Can you work these out from the model? Positions are in its coordinate system, mm. Face numbers are marked on the shaded views. A direction names the side the tool comes from. Give positions to 0.01 mm unless a question says otherwise; leave off trailing zeros. Loops run counter-clockwise (first coordinate to the right, second up) from the corner with the lowest first, then second, coordinate; pieces in that order, holes last.
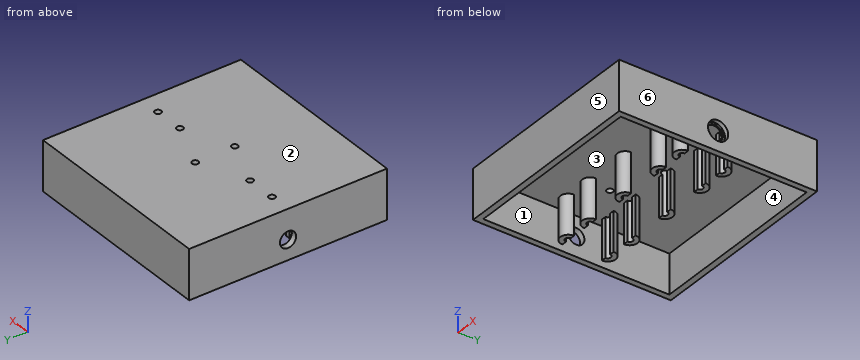
from build123d import *

# Parameters (mm, degrees)
F0_W           = 100
F0_H           = 100
F1_DEPTH       = 25
F2_W           = 94
F2_H           = 94
F3_DEPTH       = 20
F5_D           = 8.2
F5_CBORE_D     = 10.2
F5_CBORE_DEPTH = 2.2
F6_R           = 4
F7_DEPTH       = 25
F9_D           = 3.2
F10_R          = 1.6
F11_DEPTH      = 20
F12_W          = 94
F12_H          = 20
F13_DEPTH      = 20


with BuildPart() as f1:
    # F0 (on Top) → F1 (new body)
    with BuildSketch(Plane.XY):
        Rectangle(F0_W, F0_H)
    extrude(amount=F1_DEPTH)

    # F2 (on Top) → F3 (cut)
    with BuildSketch(Plane.XY):
        Rectangle(F2_W, F2_H)
    extrude(amount=F3_DEPTH, mode=Mode.SUBTRACT)

    # F5 (through all)
    with Locations(Plane.YZ.offset(50)):
        with Locations((0, 10)):
            CounterBoreHole(F5_D / 2, F5_CBORE_D / 2, F5_CBORE_DEPTH)

    # F6 (on face) → F7 (join)
    with BuildSketch(Plane.XY.offset(25)):
        with Locations((0, -10)):
            Circle(F6_R)
        with Locations((0, 10)):
            Circle(F6_R)
        with Locations((-24, 10)):
            Circle(F6_R)
        with Locations((-39, 10)):
            Circle(F6_R)
        with Locations((24, 10)):
            Circle(F6_R)
        with Locations((39, 10)):
            Circle(F6_R)
        with Locations((-24, -10)):
            Circle(F6_R)
        with Locations((24, -10)):
            Circle(F6_R)
        with Locations((39, -10)):
            Circle(F6_R)
        with Locations((-39, -10)):
            Circle(F6_R)
    extrude(amount=-F7_DEPTH)

    # F9 (through all)
    with Locations(Plane.XY.offset(25)):
        with Locations((-39, 0), (-24, 0), (0, 10), (24, 0), (39, 0), (0, -10)):
            Hole(F9_D / 2)

    # F10 (on Top) → F11 (cut)
    with BuildSketch(Plane.XY):
        with Locations((-39, -10)):
            Circle(F10_R)
        with Locations((-24, -10)):
            Circle(F10_R)
        with Locations((-24, 10)):
            Circle(F10_R)
        with Locations((-39, 10)):
            Circle(F10_R)
        with Locations((24, 10)):
            Circle(F10_R)
        with Locations((39, 10)):
            Circle(F10_R)
        with Locations((39, -10)):
            Circle(F10_R)
        with Locations((24, -10)):
            Circle(F10_R)
    extrude(amount=F11_DEPTH, mode=Mode.SUBTRACT)

    # F12 (on Top) → F13 (cut)
    with BuildSketch(Plane.XY):
        Rectangle(F12_W, F12_H)
    extrude(amount=F13_DEPTH, mode=Mode.SUBTRACT)


solid = f1.part
(1) Thinking about a two-plate mould opening in X: for the marked faces 3, 4, 5 and 6, which applies, pulls with the +X half, pulls with the -X half, needs draft (parallel to the pull), parting line crosses it, or undercut?
Returned:
face 3: undercut
face 4: undercut
face 5: needs draft
face 6: pulls with the +X half
(2) Suppose I cut it at A-A on x = -39. List the corners of the cut face in (y, z) for me, plus the area to 3 significant figures.
Returned:
outline: (-50, 0) - (-47, 0) - (-47, 20) - (-14, 20) - (-14, 0) - (-11.6, 0) - (-11.6, 20) - (-1.6, 20) - (-1.6, 25) - (-50, 25) - close; (1.6, 20) - (11.6, 20) - (11.6, 0) - (14, 0) - (14, 20) - (47, 20) - (47, 0) - (50, 0) - (50, 25) - (1.6, 25) - close
area: 700 mm2
(3) Suppose I cut it at D-D on x = 0. List the corners of the cut face in (y, z) for me, plus the area to 3 significant figures.
Returned:
outline: (-50, 0) - (-47, 0) - (-47, 20) - (-14, 20) - (-14, 0) - (-11.6, 0) - (-11.6, 25) - (-50, 25) - close; (-8.4, 20) - (8.4, 20) - (8.4, 25) - (-8.4, 25) - close; (11.6, 0) - (14, 0) - (14, 20) - (47, 20) - (47, 0) - (50, 0) - (50, 25) - (11.6, 25) - close
area: 684 mm2
(4) Which directions (+Z, -Z, +X, -X, +Y, -Y) give clear straight access to the entire face, cutting with the end or side of a thin tool? Please do the marked faces 1 and 2.
Returned:
face 1: -Z
face 2: +Z, +X, -X, +Y, -Y
(5) Will these pins go through, and if not, where does the flat tip stop? P1, Ø12, axis at x = 26, y = 23, coming from the -Z side; P2, Ø2.5, axis at x = 24, y = 0, coming from the +Z side; P3, Ø9.5, axis at y = 0, z = 10, coming from the +X side.
Returned:
P1: stops at z = 20
P2: passes through
P3: stops at x = 47.8
(6) Please list where these lines run through material, in increasing order: probe 1 along Y at (x, z) = (0, 10.25); probe 2 along Y at (x, z) = (17.5, 12.5).
Returned:
probe 1: y = -50 to -47, -14 to -11.6, 11.6 to 14, 47 to 50
probe 2: y = -50 to -47, 47 to 50
(7) Suppose I cut it at C-C on z = 17.5. Give the number of separate pieces and of enclosed holes in the cut face, plus the area to 3 significant figures.
Returned:
separate pieces: 11
enclosed holes: 1
area: 1,380 mm2
(8) Suppose I cut it at B-B on y = 44. List the corners of the cut face in (x, z) for me.
Returned:
outline: (-50, 0) - (-47, 0) - (-47, 20) - (47, 20) - (47, 0) - (50, 0) - (50, 25) - (-50, 25) - close
